For this review, take the finished solid that the model builds, in its own axes (mm). A direction names the side the tool comes from. Coordinates: 2 decimals unless noted, no trailing zeros. Order: outer loops, then holes, each group sorted by start corner. A loop starts at its lowest first (then second) coordinate and runs counter-clockwise, first axis right, second up.
from build123d import *

# Parameters (mm, degrees)
SKETCH1_W           = 39
SKETCH1_H           = 40
BOSS_EXTRUDE1_DEPTH = 18.7
SKETCH2_R           = 2
CUT_EXTRUDE1_DEPTH  = 3
SKETCH3_R           = 6.417093559
BOSS_EXTRUDE4_DEPTH = 27


with BuildPart() as part:
    # Sketch1 → Boss-Extrude1 (new body)
    with BuildSketch(Plane(origin=(0, 0, 0), x_dir=(1, 0, 0), z_dir=(0, 1, 0))):
        with Locations((19.5, 20)):
            Rectangle(SKETCH1_W, SKETCH1_H)
    extrude(amount=BOSS_EXTRUDE1_DEPTH)

    # Sketch2 → Cut-Extrude1 (cut)
    with BuildSketch(Plane(origin=(0, 18.7, 0), x_dir=(1, 0, 0), z_dir=(0, 1, 0))):
        with Locations((2.5, 14)):
            Circle(SKETCH2_R)
        with Locations((36.5, 14)):
            Circle(SKETCH2_R)
        with Locations((19.5, 33)):
            Circle(SKETCH2_R)
    extrude(amount=-CUT_EXTRUDE1_DEPTH, mode=Mode.SUBTRACT)

    # Sketch3 → Boss-Extrude4 (add)
    with BuildSketch(Plane(origin=(0, 0, -40), x_dir=(-1, 0, 0), z_dir=(0, 0, -1))):
        with Locations((-32.458546779, 9.35)):
            Circle(SKETCH3_R)
        with Locations((-19.5, 9.35)):
            Circle(SKETCH3_R)
        with Locations((-6.541453221, 9.35)):
            Circle(SKETCH3_R)
    extrude(amount=BOSS_EXTRUDE4_DEPTH)


solid = part.part
1. Take a section at A-A, the plane x = 19.5. Give the boundary of the cut face in (y, z), plus the area to 3 significant figures.
Answer below:
outline: (0, -40) - (2.93, -40) - (2.93, -67) - (15.77, -67) - (15.77, -40) - (18.7, -40) - (18.7, -35) - (15.7, -35) - (15.7, -31) - (18.7, -31) - (18.7, 0) - (0, 0) - close
area: 1,080 mm2
2. To check wall thickness, follow L1, parallel to X at y = 16.5, z = -14; L2, parallel to Z at x = 2.5, y = 16.85; L3, parallel to X at y = 18, z = -33. State the ranges of each line that lie inside material, in increasing order.
Answer below:
L1: x = 0 to 0.5, 4.5 to 34.5, 38.5 to 39
L2: z = -40 to -16, -12 to 0
L3: x = 0 to 17.5, 21.5 to 39
3. Take a section at B-B, the plane z = -14. Give the boundary of the cut face in (x, y), plus the area to 3 significant figures.
Answer below:
outline: (0, 0) - (39, 0) - (39, 18.7) - (38.5, 18.7) - (38.5, 15.7) - (34.5, 15.7) - (34.5, 18.7) - (4.5, 18.7) - (4.5, 15.7) - (0.5, 15.7) - (0.5, 18.7) - (0, 18.7) - close
area: 705 mm2
4. Take a section at C-C, the plane y = 5.5. Give the boundary of the cut face in (x, z), plus the area to 3 significant figures.
Answer below:
outline: (0, -40) - (1.41, -40) - (1.41, -67) - (11.68, -67) - (11.68, -40) - (14.37, -40) - (14.37, -67) - (24.63, -67) - (24.63, -40) - (27.32, -40) - (27.32, -67) - (37.59, -67) - (37.59, -40) - (39, -40) - (39, 0) - (0, 0) - close
area: 2,390 mm2
5. Clearance check with flat-ended pins moving along their axes: pin 1 Ø2 at (y, z) = (15.5, -54) entering from +X; pin 2 Ø2 at (y, z) = (9, -53.5) entering from -X; pin 3 Ø1.2 at (x, z) = (20, -33) entering from +Y. State where each tip first meets the part, or that it passes through.
Answer below:
pin 1: stops at x = 36.29
pin 2: stops at x = 0.12
pin 3: stops at y = 15.7
6. Take a section at D-D, the plane z = -45. Give the boundary of the cut face in (x, y).
Answer below:
outline: circle Ø12.83 at (6.54, 9.35); circle Ø12.83 at (19.5, 9.35); circle Ø12.83 at (32.46, 9.35)
7. The part is to be moulded in two halves that separate along Z. For faces 1 (the face through (35.026, 17.221, -15.352)), 2 (the face through (0, 9, -20)), 3 (the face through (7, 9, -67)), say which applies: +Z half, -Z half, draft (parallel to the pull), parting line (faces both ways), or undercut.
Answer below:
face 1: undercut
face 2: draft
face 3: -Z half
8. Machinability: for faces 4 (the face through (33, 9, -67)), 5 (the face through (26.53, 6.89, -53.31)), 6 (the face through (2.24, 17.221, -15.983)), which of the approach directions +Z, -Z, +X, -X, +Y, -Y give a long, thin tool a straight path to every point of the face, cutting with its end or side? Answer none if there is none.
Answer below:
face 4: -Z, +X, -X, +Y, -Y
face 5: -Z
face 6: +Y
